```python
from build123d import *

# Parameters (mm, degrees)
F1_DEPTH = 20
F3_DEPTH = 10
F4_W     = 4.1598360986
F4_H     = 9.7989272326
F4_H_2   = 4.1150059551
F4_W_2   = 8.7187699974
F5_DEPTH = 12.5
F6_W     = 11.4290565252
F6_H     = 16.5465530008
F6_W_2   = 7.5056552887
F7_DEPTH = 12.5
F9_DEPTH = 10


with BuildPart() as f1:
    # F0 (on Front) → F1 (new body, symmetric)
    with BuildSketch(Plane.XZ):
        Polygon((3.9122919877, 35), (0, 0), (75.6573826075, 0), (72.7546669653, 35), (66.8505893794, 35), (61.9674493795, 14.5631379331), (29.6090823453, 35), align=None)
    extrude(amount=F1_DEPTH, both=True)

    # F2 (on Front) → F3 (cut, symmetric)
    with BuildSketch(Plane.XZ):
        with BuildLine():
            Line((44.829197228, 40.699031204), (11.7313470691, 40.699031204))
            Line((11.7313470691, 40.699031204), (11.7313470691, 22.1760364611))
            ThreePointArc((11.7313470691, 22.1760364611), (27.3392283785, 33.0721865907), (39.986979806, 18.8466310501))
            ThreePointArc((39.986979806, 18.8466310501), (38.9972583667, 13.6146205714), (36.1648645763, 9.1056264937))
            Line((36.1648645763, 9.1056264937), (44.829197228, 9.1056264937))
            Line((44.829197228, 9.1056264937), (44.829197228, 40.699031204))
        make_face()
        with BuildLine():
            ThreePointArc((39.986979806, 18.8466310501), (27.3392283785, 33.0721865907), (11.7313470691, 22.1760364611))
            Line((11.7313470691, 22.1760364611), (11.7313470691, 15.5172256391))
            ThreePointArc((11.7313470691, 15.5172256391), (13.032634994, 12.0901677157), (15.1611532505, 9.1056264937))
            Line((15.1611532505, 9.1056264937), (36.1648645763, 9.1056264937))
            ThreePointArc((36.1648645763, 9.1056264937), (38.9972583667, 13.6146205714), (39.986979806, 18.8466310501))
        make_face()
        with BuildLine():
            Line((11.7313470691, 15.5172256391), (11.7313470691, 22.1760364611))
            ThreePointArc((11.7313470691, 22.1760364611), (11.3390380208, 18.8466310501), (11.7313470691, 15.5172256391))
        make_face()
        with BuildLine():
            ThreePointArc((15.1611532505, 9.1056264937), (13.032634994, 12.0901677157), (11.7313470691, 15.5172256391))
            Line((11.7313470691, 15.5172256391), (11.7313470691, 9.1056264937))
            Line((11.7313470691, 9.1056264937), (15.1611532505, 9.1056264937))
        make_face()
        with BuildLine():
            ThreePointArc((15.1611532505, 9.1056264937), (25.6630089134, 4.5226601575), (36.1648645763, 9.1056264937))
            Line((36.1648645763, 9.1056264937), (15.1611532505, 9.1056264937))
        make_face()
    extrude(amount=F3_DEPTH, both=True, mode=Mode.SUBTRACT)

    # F4 (on Front) → F5 (cut, symmetric)
    with BuildSketch(Plane.XZ):
        with Locations((16.3239417598, 31.6951358691)):
            Rectangle(F4_W, F4_H)
        with Locations((16.3239417598, 24.7381692752)):
            Rectangle(F4_W, F4_H_2)
        with Locations((22.7632448077, 24.7381692752)):
            Rectangle(F4_W_2, F4_H_2)
    extrude(amount=F5_DEPTH, both=True, mode=Mode.SUBTRACT)

    # F6 (on Front) → F7 (cut, symmetric)
    with BuildSketch(Plane.XZ):
        with Locations((76.988093555, 34.8887415603)):
            Rectangle(F6_W, F6_H)
        with Locations((64.2796605825, 34.8887415603)):
            Rectangle(F6_W_2, F6_H)
    extrude(amount=F7_DEPTH, both=True, mode=Mode.SUBTRACT)

    # F8 (on face) → F9 (cut)
    with BuildSketch(Plane.YZ.offset(71.2735652924)):
        Polygon((-12.5068677589, 38.0216091871), (-12.5, 35), (-11.25, 32.8349364905), (-10, 35), (-8.75, 32.8349364905), (-7.5, 35), (-6.25, 32.8349364905), (-5, 35), (-3.75, 32.8349364905), (-2.5, 35), (-1.25, 32.8349364905), (0, 35), (1.25, 32.8349364905), (2.5, 35), (3.75, 32.8349364905), (5, 35), (6.25, 32.8349364905), (7.5, 35), (8.75, 32.8349364905), (10, 35), (11.25, 32.8349364905), (12.5, 35), (12.5, 38.0216091871), align=None)
    extrude(amount=-F9_DEPTH, mode=Mode.SUBTRACT)


solid = f1.part
```
Could you check a few things on this model? Use its own coordinates, in mm. A direction names the side the tool comes from. Round coordinates to 2 decimals unless told otherwise and drop trailing zeros. Loops run counter-clockwise (first coordinate to the right, second up) from the corner with the lowest first, then second, coordinate; pieces in that order, holes last. Notation, with made-up numbers: M 33.5,16.25 L 77.5,16.25 A26 cw 77.5,37.25 Z; hole C -0.5,64.25 d8. An arc over 180 degrees is marked long. Put each result on its own line as item: value.
Q1. Imagine slicing it at B-B (z = 30.5). Write out the boundary of the cut face in (x, y), then the cut area to 3 significant figures.
Check result:
outline: M 3.41,-20 L 36.73,-20 L 36.73,-10 L 18.4,-10 L 18.4,-12.5 L 14.24,-12.5 L 14.24,-10 L 11.73,-10 L 11.73,10 L 14.24,10 L 14.24,12.5 L 18.4,12.5 L 18.4,10 L 36.73,10 L 36.73,20 L 3.41,20 Z; M 65.78,-20 L 73.13,-20 L 73.13,-12.5 L 71.27,-12.5 L 71.27,12.5 L 73.13,12.5 L 73.13,20 L 65.78,20 L 65.78,12.5 L 68.03,12.5 L 68.03,-12.5 L 65.78,-12.5 Z
area: 1,000 mm2
Q2. Imagine slicing it at C-C (y = 14.5). Write out the boundary of the cut face in (x, z), then the cut area to 3 significant figures.
Check result:
outline: M 0,0 L 75.66,0 L 72.75,35 L 66.85,35 L 61.97,14.56 L 29.61,35 L 3.91,35 Z
area: 2,150 mm2
Q3. Imagine slicing it at D-D (x = 69.5). Write out the boundary of the cut face in (y, z).
Check result:
outline: M -20,0 L 20,0 L 20,35 L 12.5,35 L 11.25,32.83 L 10,35 L 8.75,32.83 L 7.5,35 L 6.25,32.83 L 5,35 L 3.75,32.83 L 2.5,35 L 1.25,32.83 L 0,35 L -1.25,32.83 L -2.5,35 L -3.75,32.83 L -5,35 L -6.25,32.83 L -7.5,35 L -8.75,32.83 L -10,35 L -11.25,32.83 L -12.5,35 L -20,35 Z
Q4. Thinking about a two-plate mould opening in X: for faces 1 (the face through (70, -16, 35)), 2 (the face through (1.984, -0.28, 17.745)), 3 (the face through (11.34, -0.14, 18.89)), which applies, released by +X, released by -X, zero draft, split by the parting line, or undercut?
Check result:
face 1: zero draft
face 2: released by -X
face 3: undercut
Q5. Imagine slicing it at A-A (z = 20.5). Write out the boundary of the cut face in (x, y), then the cut area to 3 significant figures.
Check result:
outline: M 2.29,-20 L 52.57,-20 L 52.57,20 L 2.29,20 Z; M 63.39,-20 L 73.96,-20 L 73.96,20 L 63.39,20 Z; hole M 11.43,-10 L 44.83,-10 L 44.83,10 L 11.43,10 Z
area: 1,770 mm2
Q6. I need wall thicknesses on probe 1 along Y at (x, z) = (36.5, 22); probe 2 along X at (y, z) = (-9.5, 15.5); probe 3 along Z at (x, y) = (25, -10.5). Which ranges of each line are inside material? Lowest first, please.
Check result:
probe 1: -20 to -10, 10 to 20
probe 2: 1.73 to 11.73, 44.83 to 60.48, 62.19 to 74.37
probe 3: 0 to 22.68, 26.8 to 35
Q7. On a 3-axis mill with a long thin cutter (end or side, diameter ignored), from which of +Z, -Z, +X, -X, +Y, -Y can I reach the whole of each face in a straight line? I mean faces 4 (the face through (72, 0, 26.615)), 5 (the face through (21, 11, 22.681)), 6 (the face through (67, -12.5, 30)). Say none if no direction works.
Check result:
face 4: +Z, +X
face 5: none
face 6: +Z
Q8. For pin 1 (1.2 mm diameter, centred on y = -11.5, z = 30.5, fed in from -X); pin 2 (0.8 mm diameter, centred on x = 24.5, y = -12, fed in from -Z); pin 3 (1.5 mm diameter, centred on y = 0.5, z = 31, fed in from -X); pin 4 (3.5 mm diameter, centred on x = 66, y = 3, fed in from +Z), each with a flat end and sliding along its axis, tell me the tip position at first contact or that it passes through.
Check result:
pin 1: x = 3.34
pin 2: z = 0
pin 3: x = 3.38
pin 4: z = 26.62
